Could you check a few things on this model? Use its own coordinates, in mm. A direction names the side the tool comes from. Give positions to 0.01 mm unless a question says otherwise; leave off trailing zeros. Loops run counter-clockwise (first coordinate to the right, second up) from the corner with the lowest first, then second, coordinate; pieces in that order, holes last. Notation, with made-up numbers: M -2.5,82 L 38.5,82 A29 cw 38.5,113 Z; hole C 69,-2 d6. An arc over 180 degrees is marked long. Answer in a Markdown table with one row per item. Add a question column.
```python
from build123d import *

# Parameters (mm, degrees)
SKETCH1_W           = 71
SKETCH1_H           = 29.5
SKETCH1_W_2         = 16
SKETCH1_H_2         = 12
BOSS_EXTRUDE2_DEPTH = 2
BOSS_EXTRUDE3_DEPTH = 17.1
SKETCH3_W           = 16
SKETCH3_H           = 7
CUT_EXTRUDE1_DEPTH  = 50.953077983
CHAMFER1_SIZE       = 2
BOSS_EXTRUDE4_DEPTH = 11
SKETCH8_R           = 1.15
CUT_EXTRUDE3_DEPTH  = 43.925778968
SKETCH9_R           = 2.175
CUT_EXTRUDE4_DEPTH  = 11.5


with BuildPart() as part:
    # Sketch1 → Boss-Extrude2 (new body)
    with BuildSketch(Plane.XY):
        Rectangle(SKETCH1_W, SKETCH1_H)
        with Locations((-14, 0)):
            Rectangle(SKETCH1_W_2, SKETCH1_H_2, mode=Mode.SUBTRACT)
    extrude(amount=BOSS_EXTRUDE2_DEPTH)

    # Sketch2 → Boss-Extrude3 (add)
    with BuildSketch(Plane.XY.offset(2)):
        Polygon((34, 13.25), (34, 4.1), (35.5, 4.1), (35.5, 14.75), (-35.5, 14.75), (-35.5, 5.25), (-34, 5.25), (-34, 13.25), align=None)
        Polygon((-34, -13.25), (34, -13.25), (34, -4.1), (35.5, -4.1), (35.5, -14.75), (-35.5, -14.75), (-35.5, -5.25), (-34, -5.25), align=None)
    extrude(amount=BOSS_EXTRUDE3_DEPTH)

    # Sketch3 → Cut-Extrude1 (cut, through all)
    with BuildSketch(Plane.XZ.offset(14.75)):
        with Locations((-14, 15.6)):
            Rectangle(SKETCH3_W, SKETCH3_H)
    extrude(amount=-CUT_EXTRUDE1_DEPTH, mode=Mode.SUBTRACT)

    # Chamfer1
    chamfer1_edges = [part.edges().sort_by_distance(p)[0] for p in [
        (-35.5, 14.75, 9.55),
        (35.5, 14.75, 9.55),
        (35.5, -14.75, 9.55),
        (-35.5, -14.75, 9.55),
    ]]
    chamfer(chamfer1_edges, length=CHAMFER1_SIZE)

    # Sketch7 → Boss-Extrude4 (add)
    with BuildSketch(Plane.XY.offset(2)):
        with BuildLine():
            Line((-34, 13.25), (-34, 7.355))
            Line((-34, 7.355), (-30.75, 7.355))
            ThreePointArc((-30.75, 7.355), (-28.85848936, 8.13848936), (-28.075, 10.03))
            Line((-28.075, 10.03), (-28, 13.25))
            Line((-28, 13.25), (-34, 13.25))
        make_face()
        with BuildLine():
            Line((34, 13.25), (28, 13.25))
            Line((28, 13.25), (28.075, 10.03))
            ThreePointArc((28.075, 10.03), (28.85848936, 8.13848936), (30.75, 7.355))
            Line((30.75, 7.355), (34, 7.355))
            Line((34, 7.355), (34, 13.25))
        make_face()
        with BuildLine():
            Line((-34, -13.25), (-28, -13.25))
            Line((-28, -13.25), (-28.075, -10.03))
            ThreePointArc((-28.075, -10.03), (-28.85848936, -8.13848936), (-30.75, -7.355))
            Line((-30.75, -7.355), (-34, -7.355))
            Line((-34, -7.355), (-34, -13.25))
        make_face()
        with BuildLine():
            Line((34, -13.25), (34, -7.355))
            Line((34, -7.355), (30.75, -7.355))
            ThreePointArc((30.75, -7.355), (28.85848936, -8.13848936), (28.075, -10.03))
            Line((28.075, -10.03), (28, -13.25))
            Line((28, -13.25), (34, -13.25))
        make_face()
    extrude(amount=BOSS_EXTRUDE4_DEPTH)

    # Sketch8 → Cut-Extrude3 (cut, through all)
    with BuildSketch(Plane(origin=(0, 0, 0), x_dir=(-1, 0, 0), z_dir=(0, 0, -1))):
        with Locations((30.75, 10.03)):
            Circle(SKETCH8_R)
        with Locations(Location((-30.75, 10.03, 0), (0, 0, 180))):
            Circle(SKETCH8_R)
        with Locations((-30.75, -10.03)):
            Circle(SKETCH8_R)
        with Locations(Location((30.75, -10.03, 0), (0, 0, 180))):
            Circle(SKETCH8_R)
    extrude(amount=-CUT_EXTRUDE3_DEPTH, mode=Mode.SUBTRACT)

    # Sketch9 → Cut-Extrude4 (cut)
    with BuildSketch(Plane(origin=(0, 0, 0), x_dir=(-1, 0, 0), z_dir=(0, 0, -1))):
        with Locations((30.75, 10.03)):
            Circle(SKETCH9_R)
        with Locations(Location((-30.75, 10.03, 0), (0, 0, 180))):
            Circle(SKETCH9_R)
        with Locations((-30.75, -10.03)):
            Circle(SKETCH9_R)
        with Locations(Location((30.75, -10.03, 0), (0, 0, 180))):
            Circle(SKETCH9_R)
    extrude(amount=-CUT_EXTRUDE4_DEPTH, mode=Mode.SUBTRACT)


solid = part.part
```
Item 1: Suppose I cut it at C-C (x = -13). List the corners of the cut face in (y, z) for me.
Item 2: For P1, Ø5, axis at x = -30.75, y = 10.03, coming from the -Z side; P2, Ø1.6, axis at y = 14, z = 15.5, coming from the -X side; P3, Ø5, axis at x = -30.75, y = -10.03, coming from the +Z side; P4, Ø1, axis at x = -5.5, y = 3.5, coming from the +Z side, each with a flat end and sliding along its axis, tell me the tip position at first contact or that it passes through.
Item 3: I need wall thicknesses on L1, parallel to Y at x = -30.75, z = 12.4 (3 decimals); L2, parallel to Y at x = 30.75, z = 4.5 (3 decimals); L3, parallel to Y at x = 12.5, z = 9.25. Which ranges of each line are inside material? Lowest first, please.
Item 4: Suppose I cut it at A-A (y = -0.75). List the corners of the cut face in (x, z) for me.
Item 5: If we mould it in two halves opening along X, with no side actions, what happens to faces 1 (the face through (-28.9, 8.1, 7.4)), 2 (the face through (-32, 7.355, 7)), 3 (the face through (0, 0, 0)), 4 (the face through (-34.49, 13.76, 9.68))? For each: +X half, -X half, draft (parallel to the pull), parting line (faces both ways), or undercut.
Item 6: For faces 5 (the face through (0, -13.25, 10)), 6 (the face through (-14, 6, 1)), 7 (the face through (35, -4.1, 10)), 8 (the face through (29.8, -11, 11.5)), 9 (the face through (-35, 5.25, 10)), which set-ups out of +Z, -Z, +X, -X, +Y, -Y let a thin tool reach every point of the face, with its end or its side?
Item 7: Suppose I cut it at B-B (z = 17). List the corners of the cut face in (x, y) for me.
Item 8: Suppose I cut it at D-D (x = 2.5). List the corners of the cut face in (y, z) for me, then the cut area to 3 significant figures.
Values found:
| question | item | result |
|---|---|---|
| 1 | outline | M -14.75,0 L -6,0 L -6,2 L -13.25,2 L -13.25,12.1 L -14.75,12.1 Z; M 6,0 L 14.75,0 L 14.75,12.1 L 13.25,12.1 L 13.25,2 L 6,2 Z |
| 2 | P1 | z = 0 |
| 2 | P2 | x = -35.05 |
| 2 | P3 | z = 13 |
| 2 | P4 | z = 2 |
| 3 | L1 | -14.75 to -11.18, -8.88 to -7.355, 7.355 to 8.88, 11.18 to 14.75 |
| 3 | L2 | -14.75 to -12.205, -7.855 to -7.355, 7.355 to 7.855, 12.205 to 14.75 |
| 3 | L3 | -14.75 to -13.25, 13.25 to 14.75 |
| 4 | outline | M -35.5,0 L -22,0 L -22,2 L -35.5,2 Z; M -6,0 L 35.5,0 L 35.5,2 L -6,2 Z |
| 5 | face 1 | undercut |
| 5 | face 2 | undercut |
| 5 | face 3 | draft |
| 5 | face 4 | -X half |
| 6 | face 5 | +Z |
| 6 | face 6 | +Z, -Z |
| 6 | face 7 | +Z, +X, -X |
| 6 | face 8 | -Z |
| 6 | face 9 | +Z, -X |
| 7 | outline | M -35.5,-12.75 L -33.5,-14.75 L -22,-14.75 L -22,-13.25 L -34,-13.25 L -34,-5.25 L -35.5,-5.25 Z; M -35.5,5.25 L -34,5.25 L -34,13.25 L -22,13.25 L -22,14.75 L -33.5,14.75 L -35.5,12.75 Z; M -6,-14.75 L 33.5,-14.75 L 35.5,-12.75 L 35.5,-4.1 L 34,-4.1 L 34,-13.25 L -6,-13.25 Z; M -6,13.25 L 34,13.25 L 34,4.1 L 35.5,4.1 L 35.5,12.75 L 33.5,14.75 L -6,14.75 Z |
| 8 | outline | M -14.75,0 L 14.75,0 L 14.75,19.1 L 13.25,19.1 L 13.25,2 L -13.25,2 L -13.25,19.1 L -14.75,19.1 Z |
| 8 | area | 110 mm² |
